Check sheet for the modelled part. Datum: model origin and axes. Units: mm. Face numbers are marked on the shaded views. A direction names the side the tool comes from. Round coordinates to 2 decimals unless told otherwise and drop trailing zeros. Loops run counter-clockwise (first coordinate to the right, second up) from the corner with the lowest first, then second, coordinate; pieces in that order, holes last. Notation, with made-up numbers: (37, 35) -> (78, 35) arc R22 cw to (78, 48) -> close; hole circle Ø7 at (-35, 86.5). An arc over 180 degrees is marked (long way). Return JSON: item names as keys, results as strings.
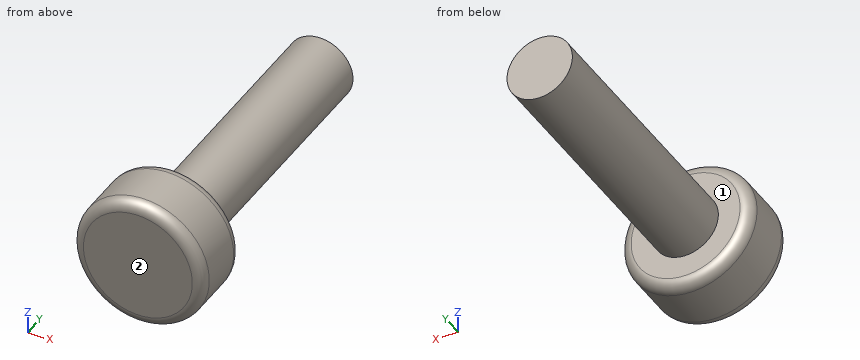
Autodesk Inventor part; units mm, degrees
ref_plane "YZ Plane" through (0, 0, 0) normal (1, 0, 0) x (0, 1, 0)
ref_plane "XZ Plane" through (0, 0, 0) normal (0, 1, 0) x (-1, 0, 0)
ref_plane "XY Plane" through (0, 0, 0) normal (0, 0, 1) x (1, 0, 0)
sketch "Sketch1" plane through (0, 0, 0) normal (0, 1, 0) x (-1, 0, 0)
  circle A0 centre (0, 0) radius 3
  dimension "d0" = 6
extrude "Extrusion1" add sketch "Sketch1" along normal blind 3
sketch "Sketch2" plane through (0, 3, 0) normal (0, 1, 0) x (1, 0, 0)
  circle A0 centre (0, 0) radius 1.5
  dimension "d3" = 3
extrude "Extrusion2" add sketch "Sketch2" along normal blind 12
fillet "Fillet1" radius 0.5 2 edges at (3, 3, 0) (3, 0, 0)
thread "Thread1"
properties part number "M3_12mm"
Q1. Section check C-C (y = 4.5). Record the boundary of the cut face in (x, z).
Results list:
{"outline": "circle Ø3 at (0, 0)"}
Q2. Material ranges on line 1 (Y direction, x = 1.45, z = -2.1); line 2 (X direction, y = 5.25, z = -1.1); line 3 (Z direction, x = 1.25, y = 12), recorded low to high.
Results list:
{"line 1": "0 to 3", "line 2": "-1.02 to 1.02", "line 3": "-0.83 to 0.83"}
Q3. Section check B-B (x = 0). Record the boundary of the cut face in (y, z).
Results list:
{"outline": "(0, -2.5) arc R0.5 ccw to (0.5, -3) -> (2.5, -3) arc R0.5 ccw to (3, -2.5) -> (3, -1.5) -> (15, -1.5) -> (15, 1.5) -> (3, 1.5) -> (3, 2.5) arc R0.5 ccw to (2.5, 3) -> (0.5, 3) arc R0.5 ccw to (0, 2.5) -> close"}
Q4. Section check A-A (z = 0). Record the boundary of the cut face in (x, y).
Results list:
{"outline": "(-3, 0.5) arc R0.5 ccw to (-2.5, 0) -> (2.5, 0) arc R0.5 ccw to (3, 0.5) -> (3, 2.5) arc R0.5 ccw to (2.5, 3) -> (1.5, 3) -> (1.5, 15) -> (-1.5, 15) -> (-1.5, 3) -> (-2.5, 3) arc R0.5 ccw to (-3, 2.5) -> close"}
Q5. Go/stop test with flat-tipped pins: pin 1 (3 mm diameter, centred on y = 10.5, z = 2, fed in from -X); pin 2 (3 mm diameter, centred on x = 0, z = -2, fed in from -Y); pin 3 (1.5 mm diameter, centred on x = -1.5, y = 6.5, fed in from -Z). Record where each tip stops, or that it passes through.
Results list:
{"pin 1": "x = -1.41", "pin 2": "y = 0", "pin 3": "z = -1.3"}
Q6. Tool access check on the marked faces 1 and 2. Record the directions out of +Z, -Z, +X, -X, +Y, -Y that give a thin tool (end or side, any length) a straight path to the whole face; none if there is none.
Results list:
{"face 1": "+Y", "face 2": "+Z, -Z, +X, -X, -Y"}
